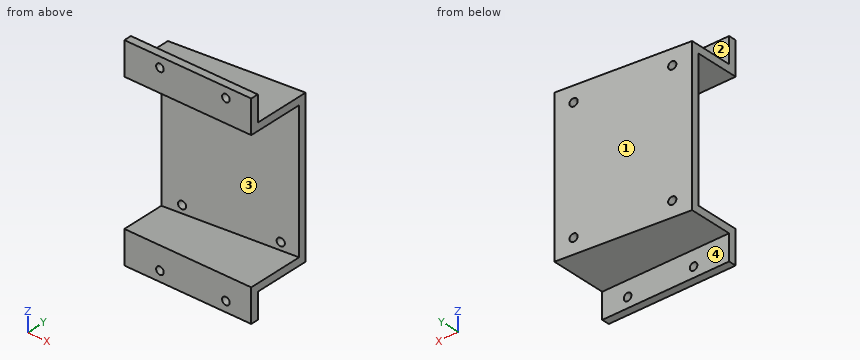
```python
from build123d import *

# Parameters (mm, degrees)
EXTRUDE_3_DEPTH     = 3
EXTRUDE_4_DEPTH     = 54
EXTRUDE_5_DEPTH     = 3
SKETCH_9_W          = 50
SKETCH_9_H          = 3
EXTRUDE_6_DEPTH     = 10
SKETCH_10_W         = 50
SKETCH_10_H         = 3
EXTRUDE_7_DEPTH     = 10
SKETCH_11_R         = 1.5
CUT_EXTRUDE_1_DEPTH = 7
SKETCH_12_R         = 1.5
CUT_EXTRUDE_2_DEPTH = 7


with BuildPart() as part:
    # 草图4 → 凸台-拉伸3 (new body)
    with BuildSketch(Plane.XY):
        Polygon((0, 0), (50, 0), (50, 25), (0, 20), align=None)
    extrude(amount=EXTRUDE_3_DEPTH)

    # 草图5 → 凸台-拉伸4 (add)
    with BuildSketch(Plane.XY.offset(3)):
        Polygon((0, 20), (0, 17), (50, 22), (50, 25), align=None)
    extrude(amount=EXTRUDE_4_DEPTH)

    # 草图8 → 凸台-拉伸5 (add)
    with BuildSketch(Plane.XY.offset(57)):
        Polygon((0, 20), (50, 25), (50, 0), (0, 0), align=None)
    extrude(amount=EXTRUDE_5_DEPTH)

    # 草图9 → 凸台-拉伸6 (add)
    with BuildSketch(Plane.XY.offset(60)):
        with Locations((25, 1.5)):
            Rectangle(SKETCH_9_W, SKETCH_9_H)
    extrude(amount=EXTRUDE_6_DEPTH)

    # 草图10 → 凸台-拉伸7 (add)
    with BuildSketch(Plane(origin=(0, 0, 0), x_dir=(-1, 0, 0), z_dir=(0, 0, -1))):
        with Locations((-25, 1.5)):
            Rectangle(SKETCH_10_W, SKETCH_10_H)
    extrude(amount=EXTRUDE_7_DEPTH)

    # 草图11 → 切除-拉伸1 (cut)
    with BuildSketch(Plane(origin=(0, 3, 0), x_dir=(1, 0, 0), z_dir=(0, 1, 0))):
        with Locations(Location((14, -66, 0), (0, 0, 270))):
            Circle(SKETCH_11_R)
        with Locations(Location((40, -66, 0), (0, 0, 270))):
            Circle(SKETCH_11_R)
        with Locations(Location((40, 6, 0), (0, 0, 270))):
            Circle(SKETCH_11_R)
        with Locations(Location((14, 6, 0), (0, 0, 270))):
            Circle(SKETCH_11_R)
    extrude(amount=-CUT_EXTRUDE_1_DEPTH, mode=Mode.SUBTRACT)

    # 草图12 → 切除-拉伸2 (cut)
    with BuildSketch(Plane(origin=(-1.98019802, 19.801980198, 0), x_dir=(0.9950371902099892, 0.09950371902099896, 0), z_dir=(-0.09950371902099897, 0.9950371902099893, 0))):
        with Locations(Location((45.239452486, -6, 0), (0, 0, 180))):
            Circle(SKETCH_12_R)
        with Locations(Location((45.239452486, -54, 0), (0, 0, 180))):
            Circle(SKETCH_12_R)
        with Locations(Location((9.239452486, -54, 0), (0, 0, 180))):
            Circle(SKETCH_12_R)
        with Locations(Location((9.239452486, -6, 0), (0, 0, 180))):
            Circle(SKETCH_12_R)
    extrude(amount=-CUT_EXTRUDE_2_DEPTH, mode=Mode.SUBTRACT)


solid = part.part
```
Verification items for the finished model (mm, model axes). Face numbers are marked on the shaded views. A direction names the side the tool comes from. Round coordinates to 2 decimals unless told otherwise and drop trailing zeros. Write each loop counter-clockwise with the first axis right and the second up, starting at its lowest first coordinate (ties: lowest second). Pieces come first, ordered by that corner, then holes. Notation, with made-up numbers: (10.5, 40.5) - (45.5, 40.5) arc R24 ccw to (45.5, 69.5) - close; hole circle Ø4 at (-12.5, -24.5). An arc over 180 degrees is marked (long way). Answer as a JSON object with one key per item and string values. Group by question number.
Q1. Thickness scan on line 1 (X direction, y = 2.3, z = -6); line 2 (Z direction, x = 38, y = 8.5); line 3 (Z direction, x = 45.5, y = 23.25). Record the ranges inside material, lowest first.
Q2. Section check D-D, the plane x = 26.5. Enter the section's corners in (y, z).
Q3. Section check B-B, the plane y = 13.25. Enter the section's corners in (x, z).
Q4. Go/stop test with flat-tipped pins: pin 1 Ø8 at (x, z) = (26.5, 55.5) entering from -Y; pin 2 Ø8 at (x, z) = (26.5, 65) entering from +Y; pin 3 Ø1.5 at (x, z) = (29, 41) entering from +Y (3 decimals); pin 4 Ø5 at (x, z) = (31, 0.5) entering from +Y. Record where each tip stops, or that it passes through.
Q5. Section check A-A, the plane x = 40. Enter the section's corners in (y, z).
Q6. Tool access check on the marked faces 1, 2, 3 and 4. Record the directions out of +Z, -Z, +X, -X, +Y, -Y that give a thin tool (end or side, any length) a straight path to the whole face; none if there is none.
Q7. Section check C-C, the plane z = -6. Enter the section's corners in (x, y), plus the area to 3 significant figures.
Found:
{
 "1": {"line 1": "x = 0 to 12.5, 15.5 to 38.5, 41.5 to 50", "line 2": "z = 0 to 3, 57 to 60", "line 3": "z = 0 to 60"},
 "2": {"outline": "(0, -10) - (3, -10) - (3, 0) - (22.65, 0) - (22.65, 60) - (3, 60) - (3, 70) - (0, 70) - (0, 57) - (19.65, 57) - (19.65, 3) - (0, 3) - close"},
 "3": {"outline": "(0, 0) - (50, 0) - (50, 3) - (0, 3) - close; (0, 57) - (50, 57) - (50, 60) - (0, 60) - close"},
 "4": {"pin 1": "stops at y = 0", "pin 2": "stops at y = 3", "pin 3": "stops at y = 22.975", "pin 4": "stops at y = 23.35"},
 "5": {"outline": "(0, -10) - (3, -10) - (3, -7.5) - (0, -7.5) - close; (0, -4.5) - (3, -4.5) - (3, 0) - (24, 0) - (24, 60) - (3, 60) - (3, 64.5) - (0, 64.5) - (0, 57) - (21, 57) - (21, 3) - (0, 3) - close; (0, 67.5) - (3, 67.5) - (3, 70) - (0, 70) - close"},
 "6": {"face 1": "+Z, -Z, -X, +Y", "face 2": "+Z, +X, -X, +Y", "face 3": "+X, -Y", "face 4": "-Z, +X, -X, +Y"},
 "7": {"outline": "(0, 0) - (12.5, 0) - (12.5, 3) - (0, 3) - close; (15.5, 0) - (38.5, 0) - (38.5, 3) - (15.5, 3) - close; (41.5, 0) - (50, 0) - (50, 3) - (41.5, 3) - close", "area": "132 mm^2"}
}
